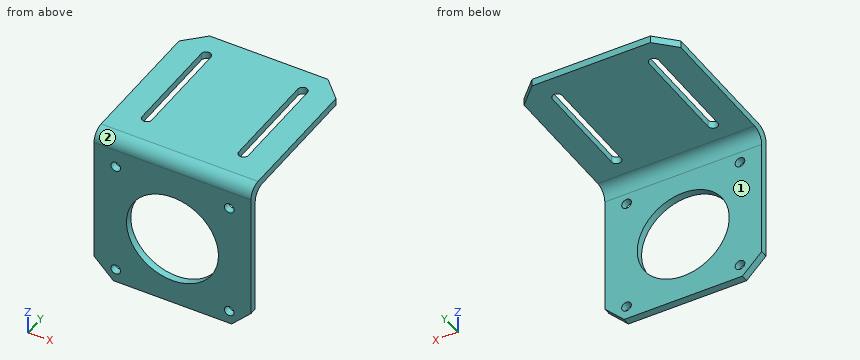
from build123d import *

# Parameters (mm, degrees)
SKETCH_2_W          = 65
SKETCH_2_H          = 65
SKETCH_2_R          = 19.05
SKETCH_2_R_2        = 2
EXTRUDE_2_DEPTH     = 3
CHAMFER_2_SIZE      = 8
SKETCH_3_W          = 65
SKETCH_3_H          = 3
EXTRUDE_3_DEPTH     = 65
FILLET_1_R          = 5
CHAMFER_3_SIZE      = 8
CUT_EXTRUDE_1_DEPTH = 65


with BuildPart() as part:
    # 草圖2 → 填料-伸長2 (new body)
    with BuildSketch(Plane(origin=(0, 0, 0), x_dir=(1, 0, 0), z_dir=(0, 1, 0))):
        Rectangle(SKETCH_2_W, SKETCH_2_H)
        with Locations((0, 3.5)):
            Circle(SKETCH_2_R, mode=Mode.SUBTRACT)
        with Locations((-23.5, 27)):
            Circle(SKETCH_2_R_2, mode=Mode.SUBTRACT)
        with Locations((-23.5, -20)):
            Circle(SKETCH_2_R_2, mode=Mode.SUBTRACT)
        with Locations((23.5, -20)):
            Circle(SKETCH_2_R_2, mode=Mode.SUBTRACT)
        with Locations((23.5, 27)):
            Circle(SKETCH_2_R_2, mode=Mode.SUBTRACT)
    extrude(amount=EXTRUDE_2_DEPTH)

    # 導角2
    chamfer_2_edges = [part.edges().sort_by_distance(p)[0] for p in [
        (-32.5, 1.5, -32.5),
        (32.5, 1.5, -32.5),
    ]]
    chamfer(chamfer_2_edges, length=CHAMFER_2_SIZE)

    # 草圖3 → 填料-伸長3 (add)
    with BuildSketch(Plane(origin=(0, 3, 0), x_dir=(1, 0, 0), z_dir=(0, 1, 0))):
        with Locations((0, -31)):
            Rectangle(SKETCH_3_W, SKETCH_3_H)
    extrude(amount=EXTRUDE_3_DEPTH)

    # 圓角1
    fillet_1_edges = [part.edges().sort_by_distance(p)[0] for p in [
        (0, 0, 32.5),
        (0, 3, 29.5),
    ]]
    fillet(fillet_1_edges, radius=FILLET_1_R)

    # 導角3
    chamfer_3_edges = [part.edges().sort_by_distance(p)[0] for p in [
        (-32.5, 68, 31),
        (32.5, 68, 31),
    ]]
    chamfer(chamfer_3_edges, length=CHAMFER_3_SIZE)

    # 草圖4 → 除料-伸長1 (cut)
    with BuildSketch(Plane(origin=(0, 0, 29.5), x_dir=(-1, 0, 0), z_dir=(0, 0, -1))):
        with BuildLine():
            Line((-18, 57.8), (-18, 16.1))
            ThreePointArc((-18, 16.1), (-20, 14.1), (-22, 16.1))
            Line((-22, 16.1), (-22, 57.8))
            ThreePointArc((-22, 57.8), (-20, 59.8), (-18, 57.8))
        make_face()
        with BuildLine():
            Line((18, 57.8), (18, 16.1))
            ThreePointArc((18, 16.1), (20, 14.1), (22, 16.1))
            Line((22, 16.1), (22, 57.8))
            ThreePointArc((22, 57.8), (20, 59.8), (18, 57.8))
        make_face()
    extrude(amount=-CUT_EXTRUDE_1_DEPTH, mode=Mode.SUBTRACT)


solid = part.part
Work out the finished part from the listing and answer in its coordinate system (mm). Face numbers are marked on the shaded views. A direction names the side the tool comes from. Give positions to 0.01 mm unless a question says otherwise; leave off trailing zeros. Order: outer loops, then holes, each group sorted by start corner. A loop starts at its lowest first (then second) coordinate and runs counter-clockwise, first axis right, second up. Notation, with made-up numbers: (85, -19) -> (136, -19) arc R21 ccw to (136, 7) -> close; hole circle Ø10 at (-36.5, 29). An arc over 180 degrees is marked (long way). One line per item, written item: value.
Item 1: Find section D-D, the plane x = -27.5. Give the vertices of the cut face in (y, z).
Answer sheet:
outline: (0, -29.5) -> (3, -29.5) -> (3, 24.5) arc R5 cw to (8, 29.5) -> (65, 29.5) -> (65, 32.5) -> (5, 32.5) arc R5 ccw to (0, 27.5) -> close
Item 2: Flat-ended cylindrical pins translate along their axes: P1, Ø5, axis at x = -17, z = 21, coming from the +Y side; P2, Ø1, axis at x = 18, z = -13.5, coming from the -Y side. Find the tip coordinate at first contact, or state that the pin passes through.
Answer sheet:
P1: y = 3
P2: y = 0
Item 3: Find section A-A, the plane z = -3.5. Give the vertices of the cut face in (x, y), plus the area to 3 significant figures.
Answer sheet:
outline: (-32.5, 0) -> (-19.05, 0) -> (-19.05, 3) -> (-32.5, 3) -> close; (19.05, 0) -> (32.5, 0) -> (32.5, 3) -> (19.05, 3) -> close
area: 80.7 mm²
Item 4: Find section C-C, the plane y = 23.5. Give the vertices of the cut face in (x, z).
Answer sheet:
outline: (-32.5, 29.5) -> (-22, 29.5) -> (-22, 32.5) -> (-32.5, 32.5) -> close; (-18, 29.5) -> (18, 29.5) -> (18, 32.5) -> (-18, 32.5) -> close; (22, 29.5) -> (32.5, 29.5) -> (32.5, 32.5) -> (22, 32.5) -> close
Item 5: Straight lines are drawn through the part: probe 1 along X at (y, z) = (1, 20); probe 2 along Z at (x, y) = (23, 1); probe 3 along X at (y, z) = (1.65, -3.5). For each, find the intervals that lie inside material, in ascending order.
Answer sheet:
probe 1: -32.5 to -25.5, -21.5 to 21.5, 25.5 to 32.5
probe 2: -32.5 to -28.94, -25.06 to 18.06, 21.94 to 30.5
probe 3: -32.5 to -19.05, 19.05 to 32.5
Item 6: A tool of negligible diameter and unlimited length cuts with its end or side. For the marked faces 1 and 2, from which of +Z, -Z, +X, -X, +Y, -Y can it reach the whole face along a straight path? Write none if from no direction.
Answer sheet:
face 1: -Z, +X, -X, +Y
face 2: +Z, +X, -X, -Y
Item 7: Find section B-B, the plane x = -20. Give the vertices of the cut face in (y, z).
Answer sheet:
outline: (0, -32.5) -> (3, -32.5) -> (3, 24.5) arc R5 cw to (8, 29.5) -> (14.1, 29.5) -> (14.1, 32.5) -> (5, 32.5) arc R5 ccw to (0, 27.5) -> close; (59.8, 29.5) -> (68, 29.5) -> (68, 32.5) -> (59.8, 32.5) -> close
